The listing builds one solid part. Answer for the finished solid, in the listing's coordinates (mm). A direction names the side the tool comes from. Give positions to 0.01 mm unless a question says otherwise; leave off trailing zeros. Write each loop counter-clockwise with the first axis right and the second up, starting at its lowest first coordinate (ties: lowest second). Pieces come first, ordered by that corner, then holes. Notation, with made-up numbers: (0.5, 5.25) -> (5.5, 5.25) arc R20 ccw to (5.5, 25.25) -> close; hole circle Ø4 at (37.25, 27). An arc over 180 degrees is marked (long way). Use CSV: the item, a comma, the result in double quotes. Start each with the question number.
from build123d import *

# Parameters (mm, degrees)
SKETCH_1_R          = 24
SKETCH_1_R_2        = 11.05
EXTRUDE_1_DEPTH     = 4
EXTRUDE_START       = -4
SKETCH_2_R          = 3
EXTRUDE_2_DEPTH     = 4
EXTRUDE_3_DEPTH     = 4
FILLET_1_R          = 2
FILLET_2_R          = 5
SKETCH_4_R          = 1.525
CUT_EXTRUDE_1_DEPTH = 4
CUT_EXTRUDE_START   = -4
CUT_EXTRUDE_2_DEPTH = 4
FILLET_3_R          = 2


with BuildPart() as part:
    # 草图1 → 凸台-拉伸1 (new body)
    with BuildSketch(Plane.XY):
        Circle(SKETCH_1_R)
        Circle(SKETCH_1_R_2, mode=Mode.SUBTRACT)
    extrude(amount=EXTRUDE_1_DEPTH)

    # 草图2 → 凸台-拉伸2 (add)
    with BuildSketch(Plane.XY.offset(4).offset(EXTRUDE_START)):
        with BuildLine():
            Line((40, 6), (23.237900077, 6))
            ThreePointArc((23.237900077, 6), (24, 0), (23.237900077, -6))
            Line((23.237900077, -6), (40, -6))
            ThreePointArc((40, -6), (46, 0), (40, 6))
        make_face()
        with Locations((40, 0)):
            Circle(SKETCH_2_R, mode=Mode.SUBTRACT)
    extrude(amount=EXTRUDE_2_DEPTH)

    # 草图3 → 凸台-拉伸3 (add)
    with BuildSketch(Plane.XY.offset(4).offset(EXTRUDE_START)):
        with BuildLine():
            Line((34.185278485, 19.927083758), (17.175, 29.74797262))
            Line((17.175, 29.74797262), (-6.485541404, 23.107093125))
            ThreePointArc((-6.485541404, 23.107093125), (11.971780948, 20.800876446), (23.237900077, 6))
            Line((23.237900077, 6), (40, 6))
            ThreePointArc((40, 6), (42.859825808, 5.274599165), (45.028144939, 3.273798783))
            Line((45.028144939, 3.273798783), (34.185278485, 19.927083758))
        make_face()
    extrude(amount=EXTRUDE_3_DEPTH)

    # 圆角1
    fillet_1_edges = [part.edges().sort_by_distance(p)[0] for p in [
        (34.185278485, 19.927083758, 2),
        (17.175, 29.74797262, 2),
    ]]
    fillet(fillet_1_edges, radius=FILLET_1_R)

    # 圆角2
    fillet_2_edges = [part.edges().sort_by_distance(p)[0] for p in [
        (23.237900077, -6, 2),
    ]]
    fillet(fillet_2_edges, radius=FILLET_2_R)

    # 草图4 → 切除-拉伸1 (cut)
    with BuildSketch(Plane.XY.offset(4)):
        with Locations((0, 20)):
            Circle(SKETCH_4_R)
        with Locations((17.320508076, 10)):
            Circle(SKETCH_4_R)
        with Locations((17.320508076, -10)):
            Circle(SKETCH_4_R)
        with Locations((0, -20)):
            Circle(SKETCH_4_R)
        with Locations((-17.320508076, -10)):
            Circle(SKETCH_4_R)
        with Locations((-17.320508076, 10)):
            Circle(SKETCH_4_R)
    extrude(amount=-CUT_EXTRUDE_1_DEPTH, mode=Mode.SUBTRACT)

    # 草图5 → 切除-拉伸2 (cut)
    with BuildSketch(Plane.XY.offset(4).offset(CUT_EXTRUDE_START)):
        with BuildLine():
            Line((8.982966985, 22.25547807), (16.498687329, 24.36493923))
            Line((16.498687329, 24.36493923), (30.648421839, 16.195586202))
            Line((30.648421839, 16.195586202), (37.057766939, 6.351634799))
            ThreePointArc((37.057766939, 6.351634799), (33.846300974, 3.336463442), (33.07179677, -1))
            Line((33.07179677, -1), (23.979157617, -1))
            ThreePointArc((23.979157617, -1), (20.170020566, 13.006547211), (8.982966985, 22.25547807))
        make_face()
    extrude(amount=CUT_EXTRUDE_2_DEPTH, mode=Mode.SUBTRACT)

    # 圆角3
    fillet_3_edges = [part.edges().sort_by_distance(p)[0] for p in [
        (23.979157617, -1, 2),
        (8.982966985, 22.25547807, 2),
        (16.498687329, 24.36493923, 2),
        (30.648421839, 16.195586202, 2),
        (37.057766939, 6.351634799, 2),
        (33.07179677, -1, 2),
    ]]
    fillet(fillet_3_edges, radius=FILLET_3_R)


solid = part.part
Q1. Section B-B on x = 25 is taken. Give the vertices of the cut face in (y, z).
Q2. Flat-ended cylindrical pins translate along their axes: pin 1 Ø1.8 at (x, y) = (17.32, 10) entering from -Z; pin 2 Ø1 at (x, z) = (-8, 2.5) entering from -Y; pin 3 Ø1 at (y, z) = (16.5, 2.5) entering from -X; pin 4 Ø1 at (x, z) = (10.5, 2) entering from -Y. Find the tip coordinate at first contact, or state that the pin passes through.
Q3. Section A-A on z = 2.3 is taken. State how many separate pieces and enclosed holes the cut face has, then the cut area to 3 significant figures.
Q4. The mould has two halves that part along Y. Classify faces 1 (the face through (17.16, 29.58, 2.03)), 2 (the face through (33.4, 11.97, 1.97)), 3 (the face through (33, -6, 2)): +Y half, -Y half, draft (parallel to the pull), parting line (faces both ways), or undercut.
Q5. Section C-C on y = 4 is taken. Give the vertices of the cut face in (x, z).
Q6. Section D-D on y = -10 is taken. Give the vertices of the cut face in (x, z).
Q7. Straight lines are drawn through the part: L1, parallel to X at y = 2.5, z = 1.5; L2, parallel to X at y = -1.5, z = 2.2; L3, parallel to Y at x = -18.5, z = 1.65. For each, find the intervals that lie inside material, in ascending order.
Q8. For faces 4 (the face through (24.58, -0.43, 2.03)), 5 (the face through (11, 9, 4)), determine the directions among +Z, -Z, +X, -X, +Y, -Y from which every point of the face is accessible in a straight line to the end or side of a thin tool.
Output:
1,outline,"(-6.35, 0) -> (-0.74, 0) -> (-0.74, 4) -> (-6.35, 4) -> close; (19.46, 0) -> (25.23, 0) -> (25.23, 4) -> (19.46, 4) -> close"
2,pin 1,"through"
2,pin 2,"y = -22.8"
2,pin 3,"x = -17.89"
2,pin 4,"y = -21.82"
3,separate pieces,"1"
3,enclosed holes,"9"
3,area,"1,780 mm²"
4,face 1,"+Y half"
4,face 2,"undercut"
4,face 3,"-Y half"
5,outline,"(-23.66, 0) -> (-10.3, 0) -> (-10.3, 4) -> (-23.66, 4) -> close; (10.3, 0) -> (23.66, 0) -> (23.66, 4) -> (10.3, 4) -> close; (34.26, 0) -> (44.56, 0) -> (44.56, 4) -> (34.26, 4) -> close"
6,outline,"(-21.82, 0) -> (-18.85, 0) -> (-18.85, 4) -> (-21.82, 4) -> close; (-15.8, 0) -> (-4.7, 0) -> (-4.7, 4) -> (-15.8, 4) -> close; (4.7, 0) -> (15.8, 0) -> (15.8, 4) -> (4.7, 4) -> close; (18.85, 0) -> (21.82, 0) -> (21.82, 4) -> (18.85, 4) -> close"
7,L1,"-23.87 to -10.76, 10.76 to 23.87, 33.46 to 38.34, 41.66 to 45.45"
7,L2,"-23.95 to -10.95, 10.95 to 37.4, 42.6 to 45.81"
7,L3,"-15.29 to -10.97, -9.03 to 9.03, 10.97 to 15.29"
8,face 4,"+Z, -Z"
8,face 5,"+Z, +X, -X, +Y, -Y"
